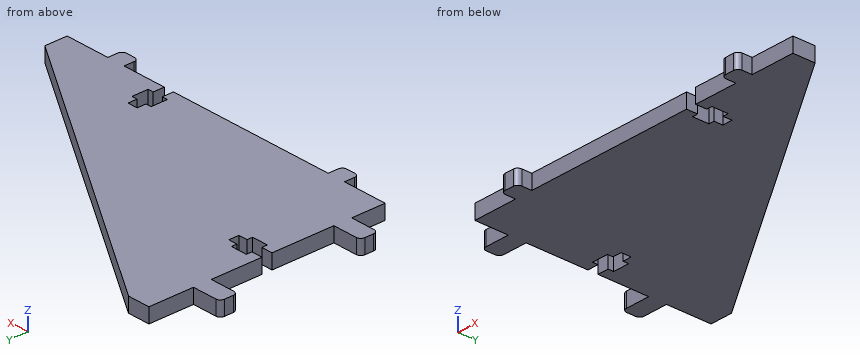
Autodesk Inventor part; units mm, degrees
ref_plane "YZ Plane" through (0, 0, 0) normal (1, 0, 0) x (0, 1, 0)
ref_plane "XZ Plane" through (0, 0, 0) normal (0, 1, 0) x (-1, 0, 0)
ref_plane "XY Plane" through (0, 0, 0) normal (0, 0, 1) x (1, 0, 0)
sketch "Sketch1" plane through (0, 0, 0) normal (0, 0, 1) x (1, 0, 0)
  line L0 (0, 106) -> (0, 0)
  line L1 (0, 0) -> (156.25, 0)
  line L2 (156.25, 0) -> (156.25, 10)
  line L3 (156.25, 10) -> (10, 106)
  line L4 (10, 106) -> (0, 106)
  dimension "d0" = 156.25
  dimension "d1" = 106
  dimension "d2" = 10
  dimension "d3" = 10
extrude "Extrusion1" add sketch "Sketch1" along normal blind 6.5
sketch "Sketch2" plane through (0, 0, 6.5) normal (0, 0, 1) x (1, 0, 0)
  line L0 (0, 106) -> (0, 0)
  line L1 (0, 0) -> (156.25, 0)
  line L2 (156.25, 0) -> (156.25, 10)
  line L3 (16.3, 55.25) -> (16.3, 50.75)
  line L4 (0, 50.75) -> (0, 55.25)
  line L5 (5, 57.75) -> (12.3, 57.75)
  line L6 (12.3, 48.25) -> (5, 48.25)
  line L7 (0, 55.25) -> (5, 55.25)
  line L8 (12.3, 55.25) -> (16.3, 55.25)
  line L9 (16.3, 50.75) -> (12.3, 50.75)
  line L10 (5, 50.75) -> (0, 50.75)
  line L11 (5, 48.25) -> (5, 50.75)
  line L12 (5, 55.25) -> (5, 57.75)
  line L13 (12.3, 57.75) -> (12.3, 55.25)
  line L14 (12.3, 50.75) -> (12.3, 48.25)
  line L15 (104, 16.3) -> (108.5, 16.3)
  line L16 (108.5, 0) -> (104, 0)
  line L17 (111, 12.3) -> (111, 5)
  line L18 (101.5, 5) -> (101.5, 12.3)
  line L19 (101.5, 12.3) -> (104, 12.3)
  line L20 (108.5, 12.3) -> (111, 12.3)
  line L21 (111, 5) -> (108.5, 5)
  line L22 (104, 5) -> (101.5, 5)
  line L23 (104, 0) -> (104, 5)
  line L24 (104, 12.3) -> (104, 16.3)
  line L25 (108.5, 16.3) -> (108.5, 12.3)
  line L26 (108.5, 5) -> (108.5, 0)
  point P0 (16.3, 53)
  point P1 (0, 53)
  point P2 (106.25, 16.3)
  dimension "d6" = 4.5
  dimension "d7" = 2.5
  dimension "d8" = 2.5
  dimension "d9" = 5
  dimension "d10" = 7.3
  dimension "d11" = 4
  dimension "d12" = 4.5
  dimension "d13" = 5
  dimension "d14" = 7.3
  dimension "d15" = 4
  dimension "d16" = 2.5
  dimension "d17" = 2.5
  dimension "d18" = 50
extrude "Extrusion2" cut sketch "Sketch2" against normal through all
sketch "Sketch3" plane through (0, 0, 6.5) normal (0, 0, 1) x (1, 0, 0)
  line L0 (0, 50.75) -> (0, 0)
  line L1 (0, 0) -> (104, 0)
  line L2 (108.5, 0) -> (156.25, 0)
  line L3 (10, 106) -> (0, 106)
  line L4 (0, 106) -> (0, 55.25)
  line L5 (0, 86) -> (-11, 86)
  line L6 (-13, 84) -> (-13, 80)
  line L7 (-11, 78) -> (0, 78)
  line L8 (0, 78) -> (0, 86)
  line L9 (0, 23) -> (-11, 23)
  line L10 (-13, 21) -> (-13, 17)
  line L11 (-11, 15) -> (0, 15)
  line L12 (0, 15) -> (0, 23)
  line L13 (20, 0) -> (28, 0)
  line L14 (28, 0) -> (28, -4.5)
  line L15 (26, -6.5) -> (22, -6.5)
  line L16 (20, -4.5) -> (20, 0)
  line L17 (128.25, 0) -> (136.25, 0)
  line L18 (136.25, 0) -> (136.25, -4.5)
  line L19 (134.25, -6.5) -> (130.25, -6.5)
  line L20 (128.25, -4.5) -> (128.25, 0)
  arc A0 (-11, 86) -> (-13, 84) centre (-11, 84) ccw
  arc A1 (-13, 80) -> (-11, 78) centre (-11, 80) ccw
  arc A2 (-11, 23) -> (-13, 21) centre (-11, 21) ccw
  arc A3 (-13, 17) -> (-11, 15) centre (-11, 17) ccw
  arc A4 (20, -4.5) -> (22, -6.5) centre (22, -4.5) ccw
  arc A5 (26, -6.5) -> (28, -4.5) centre (26, -4.5) ccw
  arc A6 (128.25, -4.5) -> (130.25, -6.5) centre (130.25, -4.5) ccw
  arc A7 (134.25, -6.5) -> (136.25, -4.5) centre (134.25, -4.5) ccw
  dimension "d21" = 2
  dimension "d22" = 8
  dimension "d23" = 8
  dimension "d24" = 8
  dimension "d25" = 8
  dimension "d26" = 13
  dimension "d27" = 6.5
  dimension "d28" = 15
  dimension "d29" = 20
  dimension "d30" = 20
  dimension "d31" = 20
extrude "Extrusion3" add sketch "Sketch3" against normal blind 6.5
properties part number "wiring_brace"
Read the model definition and answer for the solid it produces. Units are mm, in the model's axes. Round coordinates to 2 decimals unless told otherwise and drop trailing zeros. Write each loop counter-clockwise with the first axis right and the second up, starting at its lowest first coordinate (ties: lowest second). Pieces come first, ordered by that corner, then holes. Notation, with made-up numbers: (-11, -1) - (48, -1) arc R28 ccw to (48, 32) - close; hole circle Ø7 at (-26.75, 39.5). An arc over 180 degrees is marked (long way). One line per item, written item: value.
Q1. Straight lines are drawn through the part: line 1 (Y direction, x = -2.5, z = 1); line 2 (Y direction, x = 15, z = 1.25); line 3 (X direction, y = 12.5, z = 0.5). For each, find the intervals that lie inside material, in ascending order. Write a range as from..to.
The answers:
line 1: y = 15..23, 78..86
line 2: y = 0..50.75, 55.25..102.72
line 3: x = 0..104, 108.5..152.44
Q2. Each of these flat-tipped pins is pushed along its axis until it touches: P1, Ø1, axis at y = 9.5, z = 4, coming from the -X side; P2, Ø3, axis at y = 78, z = 3, coming from the +X side; P3, Ø3.5, axis at y = -3.5, z = 2.5, coming from the +X side; P4, Ø4, axis at x = 9.5, y = 26, coming from the -Z side. Where does it stop, or does it pass through?
The answers:
P1: stops at x = 0
P2: stops at x = 54.94
P3: stops at x = 136.25
P4: stops at z = 0
Q3. Find section A-A (y = 2). Determine the outline of the cut face in (x, z).
The answers:
outline: (0, 0) - (104, 0) - (104, 6.5) - (0, 6.5) - close; (108.5, 0) - (156.25, 0) - (156.25, 6.5) - (108.5, 6.5) - close
Q4. Find section C-C (y = 44). Determine the outline of the cut face in (x, z).
The answers:
outline: (0, 0) - (104.45, 0) - (104.45, 6.5) - (0, 6.5) - close
Q5. Find section B-B (x = 87.5). Determine the outline of the cut face in (y, z).
The answers:
outline: (0, 0) - (55.13, 0) - (55.13, 6.5) - (0, 6.5) - close
